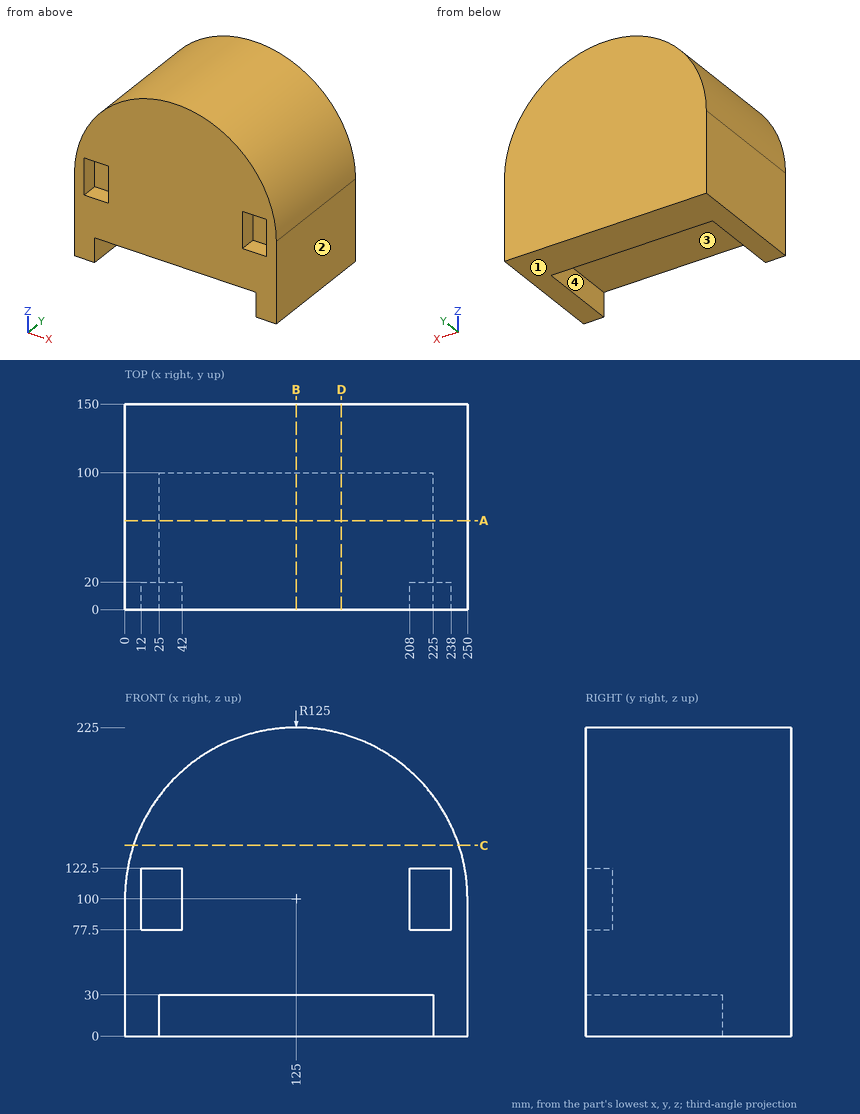
Could you check a few things on this drawing? It's one solid part, dimensions in mm from its lowest x, y, z. Give positions to 0.01 mm unless a question says otherwise; leave off trailing zeros. Order: outer loops, then holes, each group sorted by start corner. A loop starts at its lowest first (then second) coordinate and runs counter-clockwise, first axis right, second up. Notation, with made-up numbers: (-2.5, -14.5) - (12.5, -14.5) arc R22 cw to (12.5, 17.5) - close; hole circle Ø8 at (59.5, -38). An arc over 180 degrees is marked (long way). One line per item, written item: value. Start each with the question number.
1. Imagine slicing it at A-A on y = 65. List the corners of the cut face in (x, z) for me.
2. If I drill on probe 1 along Z at (x, y) = (127, 106.5); probe 2 along Y at (x, z) = (165, 22); probe 3 along Z at (x, y) = (60, 25), over which ranges is the centre line in solid material (lowest first)?
3. Imagine slicing it at C-C on z = 139. List the corners of the cut face in (x, y) for me.
4. Imagine slicing it at B-B on x = 125. List the corners of the cut face in (y, z) for me.
5. For P1, Ø3, axis at x = 206, y = 85, coming from the +Z side; P2, Ø16, axis at x = 30.5, y = 6, coming from the +Z side; P3, Ø10, axis at x = 30.5, y = 13, coming from the -Z side, each with a flat end and sliding along its axis, tell me the tip position at first contact or that it passes through.
6. Imagine slicing it at D-D on x = 158. List the corners of the cut face in (y, z) for me, plus the area to 3 significant figures.
7. Thinking about a two-plate mould opening in X: for the marked faces 1, 2, 3 and 4, which applies, +X half, -X half, draft (parallel to the pull), parting line (faces both ways), or undercut?
Values:
1. outline: (0, 0) - (25, 0) - (25, 30) - (225, 30) - (225, 0) - (250, 0) - (250, 100) arc R125 ccw to (0, 100) - close
2. probe 1: 0 to 224.98
2. probe 2: 100 to 150
2. probe 3: 30 to 206.77
3. outline: (6.24, 0) - (243.76, 0) - (243.76, 150) - (6.24, 150) - close
4. outline: (0, 30) - (100, 30) - (100, 0) - (150, 0) - (150, 225) - (0, 225) - close
5. P1: z = 196.46
5. P2: z = 190.24
5. P3: z = 30
6. outline: (0, 30) - (100, 30) - (100, 0) - (150, 0) - (150, 220.57) - (0, 220.57) - close
6. area: 30,100 mm²
7. face 1: draft
7. face 2: +X half
7. face 3: undercut
7. face 4: undercut
